Design review of the part built by this model. Coordinates are the model's own, in mm. A direction names the side the tool comes from. Coordinates: 2 decimals unless noted, no trailing zeros. Loops run counter-clockwise (first coordinate to the right, second up) from the corner with the lowest first, then second, coordinate; pieces in that order, holes last. Notation, with made-up numbers: (69, 63.25) - (106, 63.25) arc R23 cw to (106, 89.25) - close; hole circle Ø4 at (42, 24.5). An arc over 180 degrees is marked (long way). Use one line per item in the form item = value. Start each with the question number.
(1) Add section B-B (z = 15). State the section outline as (x, y) points.
(2) The part is to be moulded in two halves that separate along X. For faces 6 (the face through (0, 12, -1)), 7 (the face through (40, 16, 17)), 8 (the face through (3, 13.7, 3)), 9 (the face through (6, 15, 3)), say which applies: pulls with the +X half, pulls with the -X half, needs draft (parallel to the pull), parting line crosses it, or undercut.
(3) For L1, parallel to X at y = 14.5, z = 1.25; L2, parallel to X at y = 19.25, z = 6; L3, parallel to Z at x = 23, y = 17, list the stretches that pass through material, from the lowest coordinate up.
(4) Add section C-C (x = 47.5). State the section outline as (y, z) points, plus the area to 3 significant figures.
(5) Add section A-A (z = 1.75). State the section outline as (x, y) points, plus the area to 3 significant figures.
(6) Clearance check with flat-ended pins moving along their axes: pin 1 Ø8.5 at (x, y) = (39.5, 20.5) entering from -Z; pin 2 Ø10 at (y, z) = (18, 12.5) entering from -X; pin 3 Ø1.8 at (x, z) = (78, 3) entering from +Y. State where each tip first meets the part, or that it passes through.
(7) Add section D-D (y = 5). State the section outline as (x, z) points.
(8) Tool access review of faces 1 (the face through (51.7, 24.8, 2.4)), 2 (the face through (3, 16.3, 3)), 3 (the face through (77, 13.7, 3)), 4 (the face through (30, 16, 6)), 5 (the face through (77, 16.3, 3)): name each direction out of +Z, -Z, +X, -X, +Y, -Y from which nothing blocks a thin tool from reaching the whole face with its end or side.
```python
from build123d import *

# Parameters (mm, degrees)
SKETCH1_W           = 80
SKETCH1_H           = 4
BOSS_EXTRUDE1_DEPTH = 24.8
SKETCH2_W           = 6
SKETCH2_H           = 2.6
BOSS_EXTRUDE2_DEPTH = 6
SKETCH3_W           = 20
SKETCH3_H           = 24.8
CUT_EXTRUDE1_DEPTH  = 10
EXTRUDE_THIN1_DEPTH = 24.8
SKETCH5_W           = 20
SKETCH5_H           = 21
BOSS_EXTRUDE3_DEPTH = 7.7


with BuildPart() as part:
    # Sketch1 → Boss-Extrude1 (new body)
    with BuildSketch(Plane(origin=(0, 0, 0), x_dir=(1, 0, 0), z_dir=(0, 1, 0))):
        with Locations((40, 2)):
            Rectangle(SKETCH1_W, SKETCH1_H)
    extrude(amount=BOSS_EXTRUDE1_DEPTH)

    # Sketch2 → Boss-Extrude2 (add)
    with BuildSketch(Plane.XY):
        with Locations((3, 15)):
            Rectangle(SKETCH2_W, SKETCH2_H)
        with Locations((77, 15)):
            Rectangle(SKETCH2_W, SKETCH2_H)
    extrude(amount=BOSS_EXTRUDE2_DEPTH)

    # Sketch3 → Cut-Extrude1 (cut)
    with BuildSketch(Plane.XY):
        with Locations((40, 12.4)):
            Rectangle(SKETCH3_W, SKETCH3_H)
    extrude(amount=-CUT_EXTRUDE1_DEPTH, mode=Mode.SUBTRACT)

    # Sketch4 → Extrude-Thin1 (add)
    with BuildSketch(Plane.XZ):
        Polygon((30, 0), (30, 17), (50, 17), (50, 0), (52, 0), (52, 19), (28, 19), (28, 0), align=None)
    extrude(amount=-EXTRUDE_THIN1_DEPTH)

    # Sketch5 → Boss-Extrude3 (add)
    with BuildSketch(Plane.XZ):
        with Locations((40, 6.5)):
            Rectangle(SKETCH5_W, SKETCH5_H)
    extrude(amount=-BOSS_EXTRUDE3_DEPTH)


solid = part.part
```
Computed values:
q1.outline = (28, 0) - (52, 0) - (52, 24.8) - (50, 24.8) - (50, 7.7) - (30, 7.7) - (30, 24.8) - (28, 24.8) - close
q2.face_6 = pulls with the -X half
q2.face_7 = undercut
q2.face_8 = needs draft
q2.face_9 = undercut
q3.L1 = 0 to 6, 28 to 30, 50 to 52, 74 to 80
q3.L2 = 28 to 30, 50 to 52
q3.L3 = -4 to 0
q4.outline = (0, -4) - (7.7, -4) - (7.7, 17) - (24.8, 17) - (24.8, 19) - (0, 19) - close
q4.area = 211 mm^2
q5.outline = (0, 13.7) - (6, 13.7) - (6, 16.3) - (0, 16.3) - close; (28, 0) - (52, 0) - (52, 24.8) - (50, 24.8) - (50, 7.7) - (30, 7.7) - (30, 24.8) - (28, 24.8) - close; (74, 13.7) - (80, 13.7) - (80, 16.3) - (74, 16.3) - close
q5.area = 284 mm^2
q6.pin_1 = 17
q6.pin_2 = 28
q6.pin_3 = 16.3
q7.outline = (0, -4) - (80, -4) - (80, 0) - (52, 0) - (52, 19) - (28, 19) - (28, 0) - (0, 0) - close
q8.face_1 = +Z, -Z, +X, -X, +Y
q8.face_2 = +Z, -X, +Y
q8.face_3 = +Z, +X, -Y
q8.face_4 = -Z, +Y
q8.face_5 = +Z, +X, +Y
